Input: part model. Units: mm. Frame: model coordinates. Face numbers are marked on the shaded views. A direction names the side the tool comes from. Round coordinates to 2 decimals unless told otherwise and drop trailing zeros. Loops run counter-clockwise (first coordinate to the right, second up) from the corner with the lowest first, then second, coordinate; pieces in that order, holes last. Notation, with made-up numbers: (19.25, 59.5) -> (65.25, 59.5) arc R11 cw to (65.25, 73.5) -> close; hole circle Ø5 at (77.5, -15.75). An arc over 180 degrees is marked (long way). Answer as a JSON object with one key per item and string values.
```python
from build123d import *

# Parameters (mm, degrees)
EXTRUDE_1_DEPTH = 1.75
EXTRUDE_START   = 3
SKETCH_2_R      = 6
EXTRUDE_2_DEPTH = 3


with BuildPart() as part:
    # 草图1 → 凸台-拉伸1 (new, symmetric)
    with BuildSketch(Plane.XY):
        with BuildLine():
            Line((0, 6), (50.8, 6))
            ThreePointArc((50.8, 6), (56.8, 0), (50.8, -6))
            Line((50.8, -6), (0, -6))
            ThreePointArc((0, -6), (-6, 0), (0, 6))
        make_face()
    extrude(amount=EXTRUDE_1_DEPTH, both=True)

    # 草图2 → 凸台-拉伸2 (add)
    with BuildSketch(Plane.XY.offset(1.75).offset(EXTRUDE_START)):
        with Locations(Location((0, 0, 0), (0, 0, 270))):
            Circle(SKETCH_2_R)
    extrude(amount=-EXTRUDE_2_DEPTH)


solid = part.part
```
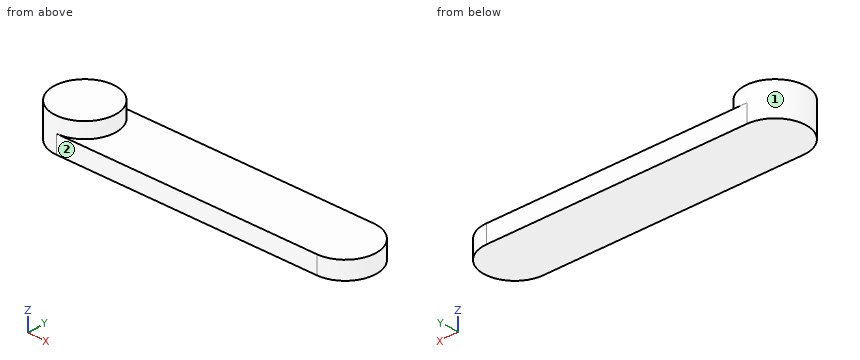
1) Section D-D, the plane y = 3.75. Output: boundary loops of the cut face in (x, z), plus the area to 3 significant figures.
Output:
{"outline": "(-4.68, -1.75) -> (55.48, -1.75) -> (55.48, 1.75) -> (4.68, 1.75) -> (4.68, 4.75) -> (-4.68, 4.75) -> close", "area": "239 mm^2"}
2) Section C-C, the plane x = 16.5. Output: boundary loops of the cut face in (y, z).
Output:
{"outline": "(-6, -1.75) -> (6, -1.75) -> (6, 1.75) -> (-6, 1.75) -> close"}
3) Contact query for flat-ended pins moving along their axis: P1, Ø1.5, axis at y = -4, z = 4, coming from the +X side; P2, Ø1, axis at y = -4.5, z = 2.5, coming from the +X side; P3, Ø2, axis at y = 4.5, z = 2, coming from the -X side. Output: stop coordinate, or through.
Output:
{"P1": "stops at x = 5.04", "P2": "stops at x = 4.47", "P3": "stops at x = -4.87"}
4) Ray query, probe 1 along Z at (x, y) = (33, 1.25); probe 2 along X at (y, z) = (-1.25, 4); probe 3 along X at (y, z) = (0.75, 3). Return the intervals inside material, ascending.
Output:
{"probe 1": "z = -1.75 to 1.75", "probe 2": "x = -5.87 to 5.87", "probe 3": "x = -5.95 to 5.95"}
5) Section A-A, the plane y = 0. Output: boundary loops of the cut face in (x, z).
Output:
{"outline": "(-6, -1.75) -> (56.8, -1.75) -> (56.8, 1.75) -> (6, 1.75) -> (6, 4.75) -> (-6, 4.75) -> close"}
6) Section B-B, the plane z = -0.25. Output: boundary loops of the cut face in (x, y), plus the area to 3 significant figures.
Output:
{"outline": "(0, -6) -> (50.8, -6) arc R6 ccw to (50.8, 6) -> (0, 6) arc R6 ccw to start", "area": "723 mm^2"}
7) Reachability of the marked faces 1 and 2 from +Z, -Z, +X, -X, +Y, -Y: full face, straight path, thin tool, end or side. Return the list, or none.
Output:
{"face 1": "+Z", "face 2": "+Z, -Z, +X, -X, -Y"}
